Read the model definition and answer for the solid it produces. Units are mm, in the model's axes. A direction names the side the tool comes from. Round coordinates to 2 decimals unless told otherwise and drop trailing zeros. Order: outer loops, then holes, each group sorted by start corner. A loop starts at its lowest first (then second) coordinate and runs counter-clockwise, first axis right, second up. Notation, with made-up numbers: M 20.5,11 L 49.5,11 A24 ccw 49.5,30 Z; hole C -23.75,17 d7. An arc over 180 degrees is marked long. Use one line per item in the form item = value. Start each with the question number.
from build123d import *

# Parameters (mm, degrees)
CROQUIS1_W                = 45
CROQUIS1_H                = 45
SALIENTE_EXTRUIR1_DEPTH   = 3
CROQUIS2_W                = 45
CROQUIS2_H                = 15
SALIENTE_EXTRUIR2_DEPTH   = 22.5
SALIENTE_EXTRUIR3_DEPTH   = 3
SIMETR_A2_COPY_1_DEPTH    = 3
CROQUIS4_R                = 2.5
CORTAR_EXTRUIR1_DEPTH     = 3
TALADRO_ROSCADO_M51_D     = 4.2
TALADRO_ROSCADO_M51_DEPTH = 18
TALADRO_ROSCADO_M51_TIP   = 1.2618073


with BuildPart() as part:
    # Croquis1 → Saliente-Extruir1 (new body)
    with BuildSketch(Plane(origin=(0, 0, 0), x_dir=(1, 0, 0), z_dir=(0, 1, 0))):
        Rectangle(CROQUIS1_W, CROQUIS1_H)
    extrude(amount=SALIENTE_EXTRUIR1_DEPTH)

    # Croquis2 → Saliente-Extruir2 (add)
    with BuildSketch(Plane(origin=(0, 3, 0), x_dir=(1, 0, 0), z_dir=(0, 1, 0))):
        Rectangle(CROQUIS2_W, CROQUIS2_H)
    extrude(amount=SALIENTE_EXTRUIR2_DEPTH)

    # Croquis3 → Saliente-Extruir3 (add)
    with BuildSketch(Plane.ZY.offset(22.5)):
        Polygon((7.5, 3), (15, 3), (7.5, 10.5), align=None)
    saliente_extruir3 = extrude(amount=-SALIENTE_EXTRUIR3_DEPTH)

    # Simetría1: Saliente-Extruir3 across plane
    add(saliente_extruir3.mirror(Plane(origin=(0, 0, 0), x_dir=(0, 0, 1), z_dir=(1, 0, 0))))

    # Simetría2: Saliente-Extruir3 across plane
    add(saliente_extruir3.mirror(Plane.XY))

    # Simetría2 copy 1 sketch → Simetría2 copy 1 (add)
    with BuildSketch(Plane(origin=(22.5, 0, 0), x_dir=(0, 0, -1), z_dir=(1, 0, 0))):
        Polygon((7.5, 3), (15, 3), (7.5, 10.5), align=None)
    extrude(amount=-SIMETR_A2_COPY_1_DEPTH)

    # Croquis4 → Cortar-Extruir1 (cut)
    with BuildSketch(Plane(origin=(0, 3, 0), x_dir=(1, 0, 0), z_dir=(0, 1, 0))):
        with Locations(Location((0, -15, 0), (0, 0, 270))):
            Circle(CROQUIS4_R)
        with Locations(Location((-12, -15, 0), (0, 0, 270))):
            Circle(CROQUIS4_R)
        with Locations(Location((12, -15, 0), (0, 0, 270))):
            Circle(CROQUIS4_R)
    cortar_extruir1 = extrude(amount=-CORTAR_EXTRUIR1_DEPTH, mode=Mode.SUBTRACT)

    # Simetría3: Cortar-Extruir1 across plane
    add(cortar_extruir1.mirror(Plane.XY), mode=Mode.SUBTRACT)

    # Taladro roscado M51
    with Locations(Plane(origin=(0, 25.5, 0), x_dir=(1, 0, 0), z_dir=(0, 1, 0))):
        with Locations((0, 0), (12, 0), (-12, 0)):
            Hole(TALADRO_ROSCADO_M51_D / 2, depth=TALADRO_ROSCADO_M51_DEPTH)
            with Locations((0, 0, -(TALADRO_ROSCADO_M51_DEPTH + TALADRO_ROSCADO_M51_TIP / 2))):  # 118° drill point
                Cone(0, TALADRO_ROSCADO_M51_D / 2, TALADRO_ROSCADO_M51_TIP, mode=Mode.SUBTRACT)


solid = part.part
Item 1: Section D-D (x = 13) is taken. Give the number of separate pieces and of enclosed holes in the cut face, and give its area (3 significant figures).
Item 2: Section A-A (y = 16) is taken. Write down the section's boundary in (x, z), and give its area (3 significant figures).
Item 3: Section C-C (z = 14) is taken. Write down the section's boundary in (x, y), and give its area (3 significant figures).
Item 4: Given P1, Ø4, axis at x = 0, z = 15, coming from the -Y side; P2, Ø4.5, axis at x = 1.5, z = -15.5, coming from the +Y side; P3, Ø4, axis at x = 8, y = 19.5, coming from the -Z side; P4, Ø2, axis at x = 4, y = 18.5, coming from the +Z side, each flat-ended and moving along its own axis, determine where each tip first touches the part or whether it passes through.
Item 5: Section B-B (x = 4.5) is taken. Write down the section's boundary in (y, z).
Item 6: A tool of negligible diameter and unlimited length cuts with its end or side. For faces 1 (the flat face through (0, 3, -18)), 2 (the cylindrical face through (14.1, 16.37, -0.09)), 3 (the flat face through (19.5, 5, 10)), from which of +Z, -Z, +X, -X, +Y, -Y can it reach the whole face along a straight path? Write none if from no direction.
Item 7: Find the intervals of material crossed by L1, parallel to X at y = 0.8, z = 15; L2, parallel to X at y = 4, z = -10; L3, parallel to Y at x = 15, z = 13, in increasing order. Write a range as [from, to].
Item 8: For a pull along X with two mould halves and no side action, classify faces 4 (the cylindrical face through (10.5, 1.5, 13)), 5 (the flat face through (-21, 7, 11)), 6 (the flat face through (-22.5, 10, 0)) as pulls with the +X half, pulls with the -X half, needs draft (parallel to the pull), parting line crosses it, or undercut.
The answers:
q1.separate_pieces = 3
q1.enclosed_holes = 0
q1.area = 377 mm²
q2.outline = M -22.5,-7.5 L 22.5,-7.5 L 22.5,7.5 L -22.5,7.5 Z; hole C -12,0 d4.2; hole C 0,0 d4.2; hole C 12,0 d4.2
q2.area = 633 mm²
q3.outline = M -22.5,0 L -14.29,0 L -14.29,3 L -19.5,3 L -19.5,4 L -22.5,4 Z; M -9.71,0 L -2.29,0 L -2.29,3 L -9.71,3 Z; M 2.29,0 L 9.71,0 L 9.71,3 L 2.29,3 Z; M 14.29,0 L 22.5,0 L 22.5,4 L 19.5,4 L 19.5,3 L 14.29,3 Z
q3.area = 99.8 mm²
q4.P1 = through
q4.P2 = 3
q4.P3 = -7.5
q4.P4 = 7.5
q5.outline = M 0,-22.5 L 3,-22.5 L 3,-7.5 L 25.5,-7.5 L 25.5,7.5 L 3,7.5 L 3,22.5 L 0,22.5 Z
q6.face_1 = -Z, +Y
q6.face_2 = +Y
q6.face_3 = +Z, +Y
q7.L1 = [-22.5, -14.5], [-9.5, -2.5], [2.5, 9.5], [14.5, 22.5]
q7.L2 = [-22.5, -19.5], [19.5, 22.5]
q7.L3 = [0, 3]
q8.face_4 = undercut
q8.face_5 = needs draft
q8.face_6 = pulls with the -X half
